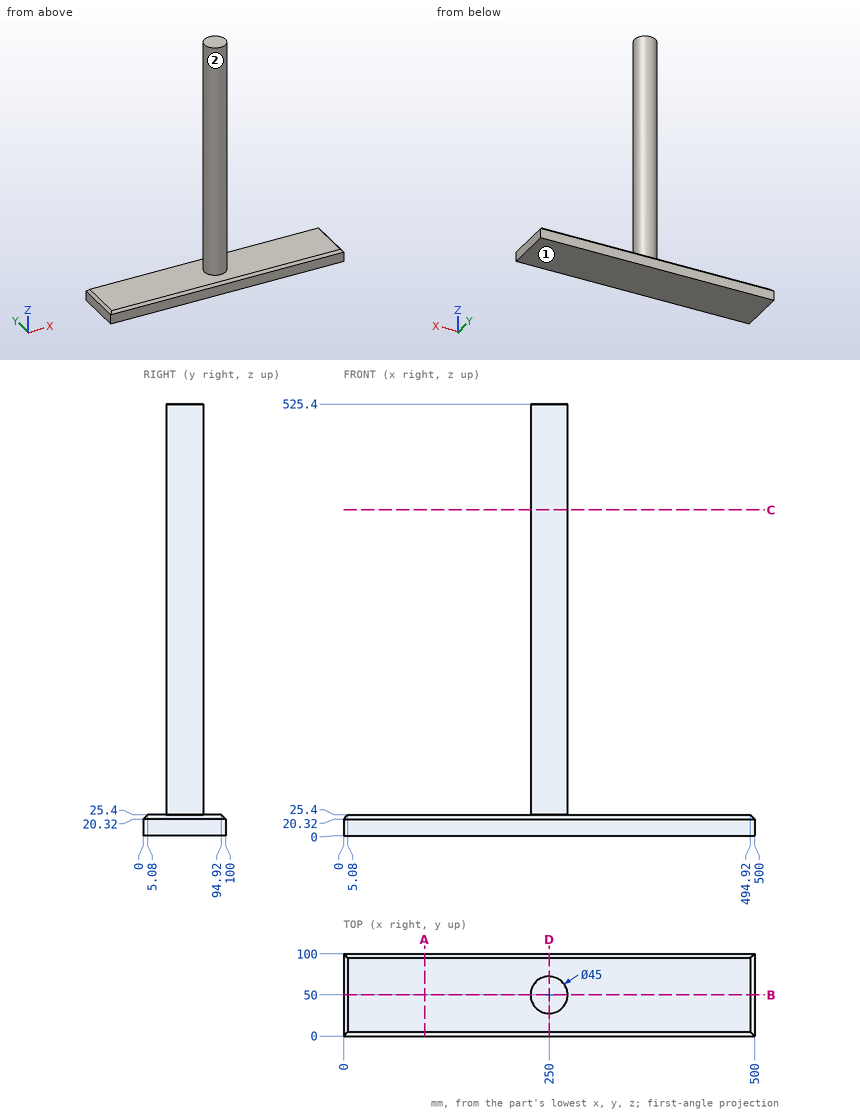
Geometry check sheet. Reference: drawing and pictorial views, mm from the part's lowest x, y, z. A direction names the side the tool comes from. Give positions to 0.01 mm unless a question says otherwise; leave off trailing zeros. Write each loop counter-clockwise with the first axis right and the second up, starting at its lowest first coordinate (ties: lowest second). Pieces come first, ordered by that corner, then holes. Notation, with made-up numbers: (59, -11) - (103, -11) arc R26 ccw to (103, 22) - close; hole circle Ø10 at (16.5, 31). An arc over 180 degrees is marked (long way). Use a Markdown table: item, result.
Q1. Section check A-A, the plane x = 98.5. Enter the section's corners in (y, z).
Computed:
| item | result |
|---|---|
| outline | (0, 0) - (100, 0) - (100, 20.32) - (94.92, 25.4) - (5.08, 25.4) - (0, 20.32) - close |
Q2. Section check D-D, the plane x = 250. Enter the section's corners in (y, z), then the cut area to 3 significant figures.
Computed:
| item | result |
|---|---|
| outline | (0, 0) - (100, 0) - (100, 20.32) - (94.92, 25.4) - (72.5, 25.4) - (72.5, 525.4) - (27.5, 525.4) - (27.5, 25.4) - (5.08, 25.4) - (0, 20.32) - close |
| area | 25,000 mm² |
Q3. Section check B-B, the plane y = 50. Enter the section's corners in (x, z), then the cut area to 3 significant figures.
Computed:
| item | result |
|---|---|
| outline | (0, 0) - (500, 0) - (500, 20.32) - (494.92, 25.4) - (272.5, 25.4) - (272.5, 525.4) - (227.5, 525.4) - (227.5, 25.4) - (5.08, 25.4) - (0, 20.32) - close |
| area | 35,200 mm² |
Q4. Section check C-C, the plane z = 396.5. Enter the section's corners in (x, y), then the cut area to 3 significant figures.
Computed:
| item | result |
|---|---|
| outline | circle Ø45 at (250, 50) |
| area | 1,590 mm² |
Q5. Go/stop test with flat-tipped pins: P1, Ø12, axis at y = 81.5, z = 228.5, coming from the +X side; P2, Ø5, axis at y = 30.5, z = 214.5, coming from the -X side; P3, Ø8, axis at x = 84.5, y = 74.5, coming from the +Z side. Record where each tip stops, or that it passes through.
Computed:
| item | result |
|---|---|
| P1 | passes through |
| P2 | stops at x = 235.26 |
| P3 | stops at z = 25.4 |
Q6. Thickness scan on L1, parallel to Z at x = 306, y = 86.5; L2, parallel to X at y = 51, z = 248.5; L3, parallel to Z at x = 143.5, y = 5. Record the ranges inside material, lowest first. Write a range as [from, to].
Computed:
| item | result |
|---|---|
| L1 | z = [0, 25.4] |
| L2 | x = [227.52, 272.48] |
| L3 | z = [0, 25.32] |
Q7. Set-up check for the marked faces 1 and 2: record each of +Z, -Z, +X, -X, +Y, -Y from which the full face is reachable in a straight line by a thin tool's end or side.
Computed:
| item | result |
|---|---|
| face 1 | -Z, +X, -X, +Y, -Y |
| face 2 | +Z |
